```python
from build123d import *

# Parameters (mm, degrees)
SKETCH1_W              = 112.659
SKETCH1_H              = 14.8813
BACKFACEPATTERN_COUNT  = 6
FRONTFACEPATTERN_COUNT = 4
SKETCH7_R              = 26.9875
SKETCH7_R_2            = 25.4
CUT_EXTRUDE1_DEPTH     = 0.5


with BuildPart() as part:
    # Sketch1 → Revolve1 (revolve)
    with BuildSketch(Plane(origin=(0, 0, 0), x_dir=(0, 0, -1), z_dir=(1, 0, 0)), mode=Mode.PRIVATE) as revolve1_sk:
        with Locations((-79.9545, 30.05935)):
            Rectangle(SKETCH1_W, SKETCH1_H)
    revolve(revolve1_sk.sketch.rotate(Axis((0, 0, 136.284), (0, 0, -1)), 90), axis=Axis((0, 0, 136.284), (0, 0, -1)))

    # Sketch9 → M6x1.0 Tapped Hole3 (revolve, cut)
    with BuildSketch(Plane(origin=(0, 31.05935, 23.625), x_dir=(0, 1, 0), z_dir=(1, 0, 0))):
        Polygon((0, 0), (0, 16.502151548), (2.5, 15), (2.5, 0), align=None)
    m6x1_0_tapped_hole3 = revolve(axis=Axis((0, 31.05935, 17.275), (0, 0, 1)), mode=Mode.SUBTRACT)

    # BackFacePattern: M6x1.0 Tapped Hole3 ×6 about axis
    backfacepattern_axis = Axis((0, 0, 0), (0, 0, 1))
    for i in range(1, BACKFACEPATTERN_COUNT):
        add(m6x1_0_tapped_hole3.rotate(backfacepattern_axis, i * 360 / BACKFACEPATTERN_COUNT), mode=Mode.SUBTRACT)

    # Sketch6 → M6x1.0 Tapped Hole2 (revolve, cut)
    with BuildSketch(Plane(origin=(0, 31.05935, 136.284), x_dir=(0, -1, 0), z_dir=(1, 0, 0))):
        Polygon((0, 0), (0, 16.502151548), (2.5, 15), (2.5, 0), align=None)
    m6x1_0_tapped_hole2 = revolve(axis=Axis((0, 31.05935, 142.634), (0, 0, -1)), mode=Mode.SUBTRACT)

    # FrontFacePattern: M6x1.0 Tapped Hole2 ×4 about axis
    frontfacepattern_axis = Axis((0, 0, 0), (0, 0, 1))
    for i in range(1, FRONTFACEPATTERN_COUNT):
        add(m6x1_0_tapped_hole2.rotate(frontfacepattern_axis, i * 360 / FRONTFACEPATTERN_COUNT), mode=Mode.SUBTRACT)

    # Sketch7 → Cut-Extrude1 (cut)
    with BuildSketch(Plane(origin=(0, 0, 23.625), x_dir=(-1, 0, 0), z_dir=(0, 0, -1))):
        with Locations(Location((0, 0, 0), (0, 0, 90))):
            Circle(SKETCH7_R)
        with Locations(Location((0, 0, 0), (0, 0, 90))):
            Circle(SKETCH7_R_2, mode=Mode.SUBTRACT)
    extrude(amount=-CUT_EXTRUDE1_DEPTH, mode=Mode.SUBTRACT)


solid = part.part
```
Check sheet for the modelled part. Datum: model origin and axes. Units: mm. A direction names the side the tool comes from. Give positions to 0.01 mm unless a question says otherwise; leave off trailing zeros. Order: outer loops, then holes, each group sorted by start corner. A loop starts at its lowest first (then second) coordinate and runs counter-clockwise, first axis right, second up. Notation, with made-up numbers: (32.5, 38) -> (42.5, 38) arc R29 cw to (42.5, 69) -> close; hole circle Ø5 at (-20.75, -3.75). An arc over 180 degrees is marked (long way). Return JSON: item names as keys, results as strings.
1. Go/stop test with flat-tipped pins: P1, Ø4, axis at x = 0, y = -31.06, coming from the -Z side; P2, Ø4.5, axis at x = 0, y = 31.06, coming from the -Z side; P3, Ø8, axis at x = 21.5, z = 70.5, coming from the -Y side; P4, Ø8, axis at x = 31.06, y = 0, coming from the +Z side. Record where each tip stops, or that it passes through.
From the geometry:
{"P1": "z = 38.93", "P2": "z = 38.77", "P3": "y = -33.17", "P4": "z = 136.28"}
2. Mould release check, pull along Y, two halves, no side actions. Record for faces 1 (the flat face through (23, 2, 23.625)), 2 (the flat face through (-16, 20, 24.125)), 3 (the cylindrical face through (17.3, 33.27, 79.17)): +Y half, -Y half, draft (parallel to the pull), parting line (faces both ways), or undercut.
From the geometry:
{"face 1": "draft", "face 2": "undercut", "face 3": "parting line"}
3. Material ranges on probe 1 along X at (y, z) = (1, 76.5); probe 2 along Y at (x, z) = (-0.5, 42); probe 3 along X at (y, z) = (32.5, 131.5), recorded low to high. Write a range as [from, to].
From the geometry:
{"probe 1": "[-37.49, -22.6], [22.6, 37.49]", "probe 2": "[-37.5, -22.61], [22.61, 37.5]", "probe 3": "[-18.71, -2.04], [2.04, 18.71]"}
4. Cross-section at D-D, the plane x = 9. Record the cut outline in (y, z) (3 decimals), plus the area to 3 significant figures.
From the geometry:
{"outline": "(-36.404, 23.625) -> (-25.443, 23.625) -> (-25.443, 24.125) -> (-23.752, 24.125) -> (-23.752, 23.625) -> (-20.751, 23.625) -> (-20.751, 136.284) -> (-36.404, 136.284) -> close; (20.751, 23.625) -> (23.752, 23.625) -> (23.752, 24.125) -> (25.443, 24.125) -> (25.443, 23.625) -> (36.404, 23.625) -> (36.404, 136.284) -> (20.751, 136.284) -> close", "area": "3,530 mm^2"}
5. Cross-section at C-C, the plane z = 115. Record the cut outline in (x, y), plus the area to 3 significant figures.
From the geometry:
{"outline": "circle Ø75 at (0, 0); hole circle Ø45.24 at (0, 0)", "area": "2,810 mm^2"}
6. Cross-section at A-A, the plane x = 20. Record the cut outline in (y, z) (3 decimals), plus the area to 3 significant figures.
From the geometry:
{"outline": "(-31.721, 23.625) -> (-18.12, 23.625) -> (-18.12, 24.125) -> (-15.658, 24.125) -> (-15.658, 23.625) -> (-10.564, 23.625) -> (-10.564, 136.284) -> (-31.721, 136.284) -> close; (10.564, 23.625) -> (15.658, 23.625) -> (15.658, 24.125) -> (18.12, 24.125) -> (18.12, 23.625) -> (31.721, 23.625) -> (31.721, 136.284) -> (10.564, 136.284) -> close", "area": "4,760 mm^2"}
7. Cross-section at B-B, the plane z = 128.5. Record the cut outline in (x, y).
From the geometry:
{"outline": "circle Ø75 at (0, 0); hole circle Ø5 at (-31.06, 0); hole circle Ø45.24 at (0, 0); hole circle Ø5 at (0, -31.06); hole circle Ø5 at (0, 31.06); hole circle Ø5 at (31.06, 0)"}
8. Set-up check for faces 4 (the flat face through (-25, 11, 23.625)), 5 (the cylindrical face through (0.11, -28.56, 31.02)), 6 (the cylindrical face through (-33.557, -0.11, 128.889)): record each of +Z, -Z, +X, -X, +Y, -Y from which the full face is reachable in a straight line by a thin tool's end or side.
From the geometry:
{"face 4": "-Z, +X, -X, +Y, -Y", "face 5": "-Z", "face 6": "+Z"}
